Could you check a few things on this model? Use its own coordinates, in mm. Coordinates: 2 decimals unless noted, no trailing zeros. Order: outer loops, then holes, each group sorted by start corner. A loop starts at its lowest first (then second) coordinate and runs counter-clockwise, first axis right, second up. Notation, with made-up numbers: (-21.5, 64) - (-7.5, 64) arc R7 cw to (-7.5, 71) - close; hole circle Ø1 at (77.25, 33). An arc over 180 degrees is marked (long way). Answer as a JSON object with one key per item and string values. Group by question number.
(1) Imagine slicing it at D-D, the plane x = -1. Write out the boundary of the cut face in (y, z), and give its area (3 significant figures).
(2) Please list where these lines run through material, in increasing order: probe 1 along Y at (x, z) = (-266, 0.35); probe 2 along Y at (x, z) = (-315, 4.55); probe 3 along Y at (x, z) = (126, 3.55).
(3) Imagine slicing it at A-A, the plane y = -225. Write out the boundary of the cut face in (x, z), and give its area (3 significant figures).
(4) Imagine slicing it at B-B, the plane x = -278. Write out the boundary of the cut face in (y, z), and give its area (3 significant figures).
(5) Imagine slicing it at C-C, the plane z = 2.8. Write out the boundary of the cut face in (x, y).
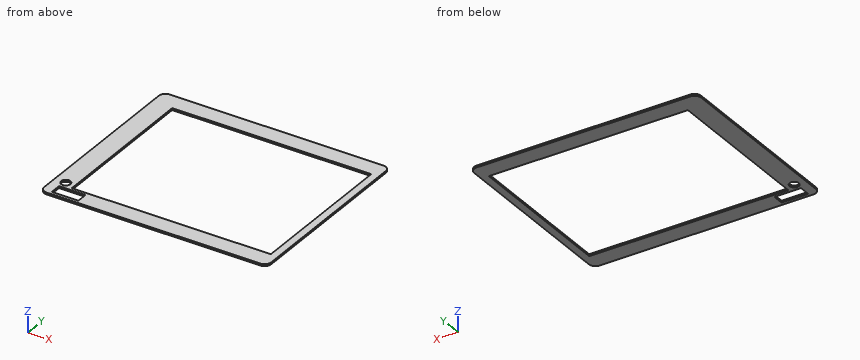
from build123d import *

# Parameters (mm, degrees)
SKETCH1_W           = 700
SKETCH1_H           = 588
BOSS_EXTRUDE1_DEPTH = 6
FILLET1_R           = 20
SKETCH2_R           = 14.4
SKETCH2_W           = 614
SKETCH2_H           = 480
SKETCH2_W_2         = 82
SKETCH2_H_2         = 34
CUT_EXTRUDE1_DEPTH  = 84


with BuildPart() as part:
    # Sketch1 → Boss-Extrude1 (new body)
    with BuildSketch(Plane.XY):
        Rectangle(SKETCH1_W, SKETCH1_H)
    extrude(amount=BOSS_EXTRUDE1_DEPTH)

    # Fillet1
    fillet1_edges = [part.edges().sort_by_distance(p)[0] for p in [
        (350, -294, 3),
        (-350, -294, 3),
        (-350, 294, 3),
        (350, 294, 3),
    ]]
    fillet(fillet1_edges, radius=FILLET1_R)

    # Sketch2 → Cut-Extrude1 (cut)
    with BuildSketch(Plane.XY.offset(6)):
        with Locations((-315, -225)):
            Circle(SKETCH2_R)
        with Locations((20, 0)):
            Rectangle(SKETCH2_W, SKETCH2_H)
        with Locations((-279.35, -266.6)):
            Rectangle(SKETCH2_W_2, SKETCH2_H_2)
    extrude(amount=-CUT_EXTRUDE1_DEPTH, mode=Mode.SUBTRACT)


solid = part.part
Result set:
{
 "1": {"outline": "(-294, 0) - (-240, 0) - (-240, 6) - (-294, 6) - close; (240, 0) - (294, 0) - (294, 6) - (240, 6) - close", "area": "648 mm^2"},
 "2": {"probe 1": "y = -294 to -283.6, -249.6 to -240, 240 to 294", "probe 2": "y = -294 to -283.6, -249.6 to -239.4, -210.6 to 294", "probe 3": "y = -294 to -240, 240 to 294"},
 "3": {"outline": "(-350, 0) - (-329.4, 0) - (-329.4, 6) - (-350, 6) - close; (-300.6, 0) - (-287, 0) - (-287, 6) - (-300.6, 6) - close; (327, 0) - (350, 0) - (350, 6) - (327, 6) - close", "area": "343 mm^2"},
 "4": {"outline": "(-294, 0) - (-283.6, 0) - (-283.6, 6) - (-294, 6) - close; (-249.6, 0) - (-240, 0) - (-240, 6) - (-249.6, 6) - close; (240, 0) - (294, 0) - (294, 6) - (240, 6) - close", "area": "444 mm^2"},
 "5": {"outline": "(-350, -274) arc R20 ccw to (-330, -294) - (330, -294) arc R20 ccw to (350, -274) - (350, 274) arc R20 ccw to (330, 294) - (-330, 294) arc R20 ccw to (-350, 274) - close; hole circle Ø28.8 at (-315, -225); hole (-320.35, -283.6) - (-238.35, -283.6) - (-238.35, -249.6) - (-320.35, -249.6) - close; hole (-287, -240) - (327, -240) - (327, 240) - (-287, 240) - close"}
}
